```python
from build123d import *

# Parameters (mm, degrees)
CYLINDER030_R         = 20.9
CYLINDER030_DEPTH     = 6
BOX007_W              = 40
BOX007_H              = 13
BOX007_DEPTH          = 5
CHAMFER009003002_SIZE = 2
CYLINDER026_R         = 2
CYLINDER026_DEPTH     = 10
CYLINDER029_R         = 2
CYLINDER029_DEPTH     = 10
CYLINDER027_R         = 2
CYLINDER027_DEPTH     = 10
BOX006_W              = 40
BOX006_H              = 4.85
BOX006_DEPTH          = 17
CHAMFER009003006_SIZE = 3
CYLINDER033_R         = 1.6
CYLINDER033_DEPTH     = 3
CYLINDER031_R         = 1.6
CYLINDER031_DEPTH     = 3
CHAMFER009003005_SIZE = 0.4
CHAMFER009003007_SIZE = 0.4


with BuildPart() as cylinder030:
    # Cylinder030 → Cylinder030 (new body)
    with BuildSketch(Plane.XY):
        Circle(CYLINDER030_R)
    extrude(amount=CYLINDER030_DEPTH)


with BuildPart() as cut004003006006002:
    # Box007 → Box007 (new body)
    with BuildSketch(Plane(origin=(-20, -25, 0), x_dir=(1, 0, 0), z_dir=(0, 0, 1))):
        with Locations((20, 6.5)):
            Rectangle(BOX007_W, BOX007_H)
    extrude(amount=BOX007_DEPTH)

    # Chamfer009003002
    chamfer009003002_edges = [cut004003006006002.edges().sort_by_distance(p)[0] for p in [
        (-20, -12, 2.5),
        (20, -12, 2.5),
    ]]
    chamfer(chamfer009003002_edges, length=CHAMFER009003002_SIZE)

    # Cut004003006006002: cut Cylinder030
    add(cylinder030.part, mode=Mode.SUBTRACT)


with BuildPart() as cylinder026:
    # Cylinder026 → Cylinder026 (new body)
    with BuildSketch(Plane(origin=(0, -20, 11), x_dir=(1, 0, 0), z_dir=(0, -1, 0))):
        Circle(CYLINDER026_R)
    extrude(amount=CYLINDER026_DEPTH)


with BuildPart() as cylinder029:
    # Cylinder029 → Cylinder029 (new body)
    with BuildSketch(Plane(origin=(15, -20, 11), x_dir=(1, 0, 0), z_dir=(0, -1, 0))):
        Circle(CYLINDER029_R)
    extrude(amount=CYLINDER029_DEPTH)


with BuildPart() as fusion001028:
    # Cylinder027 → Cylinder027 (new body)
    with BuildSketch(Plane(origin=(-15, -20, 11), x_dir=(1, 0, 0), z_dir=(0, -1, 0))):
        Circle(CYLINDER027_R)
    extrude(amount=CYLINDER027_DEPTH)

    # Fusion001028: union Cylinder026, Cylinder029
    add(cylinder026.part)
    add(cylinder029.part)


with BuildPart() as chamfer009003006:
    # Box006 → Box006 (new body)
    with BuildSketch(Plane(origin=(-20, -25, 0), x_dir=(1, 0, 0), z_dir=(0, 0, 1))):
        with Locations((20, 2.425)):
            Rectangle(BOX006_W, BOX006_H)
    extrude(amount=BOX006_DEPTH)

    # Cut004003006006003: cut Fusion001028
    add(fusion001028.part, mode=Mode.SUBTRACT)

    # Chamfer009003006
    chamfer009003006_edges = [chamfer009003006.edges().sort_by_distance(p)[0] for p in [
        (-20, -22.575, 17),
        (20, -22.575, 17),
    ]]
    chamfer(chamfer009003006_edges, length=CHAMFER009003006_SIZE)


with BuildPart() as cylinder033:
    # Cylinder033 → Cylinder033 (new body)
    with BuildSketch(Plane(origin=(16, -16, 5), x_dir=(1, 0, 0), z_dir=(0, 0, 1))):
        Circle(CYLINDER033_R)
    extrude(amount=CYLINDER033_DEPTH)


with BuildPart() as chamfer009003007:
    # Cylinder031 → Cylinder031 (new body)
    with BuildSketch(Plane(origin=(-16, -16, 5), x_dir=(1, 0, 0), z_dir=(0, 0, 1))):
        Circle(CYLINDER031_R)
    extrude(amount=CYLINDER031_DEPTH)

    # Fusion001027: union Cylinder033
    add(cylinder033.part)

    # Chamfer009003005
    chamfer009003005_edges = [chamfer009003007.edges().sort_by_distance(p)[0] for p in [
        (-17.6, -16, 8),
        (14.4, -16, 8),
    ]]
    chamfer(chamfer009003005_edges, length=CHAMFER009003005_SIZE)

    # Fusion001029: union Cut004003006006002, Chamfer009003006
    add(cut004003006006002.part)
    add(chamfer009003006.part)

    # Chamfer009003007
    chamfer009003007_edges = [chamfer009003007.edges().sort_by_distance(p)[0] for p in [
        (-18.5, -25, 15.5),
        (-17, -20.15, 11),
        (-2, -20.15, 11),
        (13, -20.15, 11),
        (18.5, -25, 15.5),
        (0, -25, 17),
        (-17, -25, 11),
        (-2, -25, 11),
        (13, -25, 11),
        (-20, -25, 7),
        (0, -25, 0),
        (20, -25, 7),
    ]]
    chamfer(chamfer009003007_edges, length=CHAMFER009003007_SIZE)


solid = chamfer009003007.part
```
CAD build for the part. Positions are in the model's coordinates, mm. A direction names the side the tool comes from. Coordinates: 2 decimals unless noted, no trailing zeros. Write each loop counter-clockwise with the first axis right and the second up, starting at its lowest first coordinate (ties: lowest second). Pieces come first, ordered by that corner, then holes. Notation, with made-up numbers: (31.25, 38.5) -> (62.25, 38.5) arc R25 cw to (62.25, 50.5) -> close; hole circle Ø1 at (51.25, 73.25). An arc over 180 degrees is marked (long way). Return JSON: item names as keys, results as strings. Group by question number.
Q1. Flat gauge pins, fed straight in: pin 1 (6.5 mm diameter, centred on x = 10.5, y = -15.5, fed in from +Z); pin 2 (1.2 mm diameter, centred on x = 16, y = -15.5, fed in from +Z); pin 3 (6.5 mm diameter, centred on x = 0, z = 11, fed in from +Y). Where does each tip first touch, or does it go through?
Q2. Cut at D-D, the plane y = -23.5. Give the cut face in (x, z).
Q3. Cut at B-B, the plane z = 6.25. Give the cut face in (x, y), then the cut area to 3 significant figures.
Q4. Drill centre lines: line 1 (X direction, y = -22.75, z = 11); line 2 (Z direction, x = -15, y = -21.4); line 3 (Y direction, x = -9.5, z = 16). Where is each one in solid material? Low to high.
Q5. Which spindle directions (+Z, -Z, +X, -X, +Y, -Y) get a long thin tool onto all of the face, cutting with end or side? Do faces 1 (the face through (15, -23, 13)), 2 (the face through (-12.123, -17.025, 2.465)), 3 (the face through (14.4, -15.93, 6.28)). Say none if no direction does.
Q6. Cut at C-C, the plane y = -16. Give the cut face in (x, z).
Q7. Pull direction X, two halves, no side cores. Call faces 4 (the face through (20, -21, 5)), 5 (the face through (11.96, -17.14, 2.46)), 6 (the face through (0, -21, 0)): released by +X, released by -X, zero draft, split by the parting line, or undercut.
Q8. Cut at A-A, the plane x = 0. Give the cut face in (y, z).
Returned:
{
 "1": {"pin 1": "stops at z = 5", "pin 2": "stops at z = 8", "pin 3": "stops at y = -20.15"},
 "2": {"outline": "(-20, 0) -> (20, 0) -> (20, 14) -> (17, 17) -> (-17, 17) -> (-20, 14) -> close; hole circle Ø4 at (-15, 11); hole circle Ø4 at (0, 11); hole circle Ø4 at (15, 11)"},
 "3": {"outline": "(-20, -24.6) -> (-19.6, -25) -> (19.6, -25) -> (20, -24.6) -> (20, -20.15) -> (-20, -20.15) -> close; circle Ø3.2 at (-16, -16); circle Ø3.2 at (16, -16)", "area": "210 mm2"},
 "4": {"line 1": "x = -20 to -17, -13 to -2, 2 to 13, 17 to 20", "line 2": "z = 0 to 9, 13 to 17", "line 3": "y = -25 to -20.15"},
 "5": {"face 1": "+Y, -Y", "face 2": "+Z, -Z, +Y", "face 3": "+Z"},
 "6": {"outline": "(-20, 0) -> (-13.45, 0) -> (-13.45, 5) -> (-14.4, 5) -> (-14.4, 7.6) -> (-14.8, 8) -> (-17.2, 8) -> (-17.6, 7.6) -> (-17.6, 5) -> (-20, 5) -> close; (13.45, 0) -> (20, 0) -> (20, 5) -> (17.6, 5) -> (17.6, 7.6) -> (17.2, 8) -> (14.8, 8) -> (14.4, 7.6) -> (14.4, 5) -> (13.45, 5) -> close"},
 "7": {"face 4": "released by +X", "face 5": "undercut", "face 6": "zero draft"},
 "8": {"outline": "(-25, 0.4) -> (-24.6, 0) -> (-20.15, 0) -> (-20.15, 8.6) -> (-20.55, 9) -> (-24.6, 9) -> (-25, 8.6) -> close; (-25, 13.4) -> (-24.6, 13) -> (-20.55, 13) -> (-20.15, 13.4) -> (-20.15, 17) -> (-24.6, 17) -> (-25, 16.6) -> close"}
}
